```python
from build123d import *

# Parameters (mm, degrees)
F0_R     = 8.05
F1_DEPTH = 3.6
F2_R     = 6
F3_DEPTH = 6
F4_R     = 8.05
F5_DEPTH = 3.1
F6_R     = 5
F7_DEPTH = 2.5
F8_R     = 2
F9_DEPTH = 15.201


with BuildPart() as f1:
    # F0 (on Top) → F1 (new body)
    with BuildSketch(Plane.XY):
        Circle(F0_R)
    extrude(amount=F1_DEPTH)

    # F2 (on face) → F3 (join)
    with BuildSketch(Plane.XY.offset(3.6)):
        Circle(F2_R)
    extrude(amount=F3_DEPTH)

    # F4 (on face) → F5 (join)
    with BuildSketch(Plane.XY.offset(9.6)):
        Circle(F4_R)
    extrude(amount=F5_DEPTH)

    # F6 (on face) → F7 (join)
    with BuildSketch(Plane.XY.offset(12.7)):
        Circle(F6_R)
    extrude(amount=F7_DEPTH)

    # F8 (on face) → F9 (cut, through all)
    with BuildSketch(Plane(origin=(0, 0, 0), x_dir=(1, 0, 0), z_dir=(0, 0, -1))):
        Circle(F8_R)
    extrude(amount=-F9_DEPTH, mode=Mode.SUBTRACT)


solid = f1.part
```
Input: part model. Units: mm. Frame: model coordinates. A direction names the side the tool comes from. Round coordinates to 2 decimals unless told otherwise and drop trailing zeros. Loops run counter-clockwise (first coordinate to the right, second up) from the corner with the lowest first, then second, coordinate; pieces in that order, holes last. Notation, with made-up numbers: (-14, 45.25) -> (42, 45.25) arc R22 cw to (42, 61.25) -> close; hole circle Ø5 at (49, -21.75). An arc over 180 degrees is marked (long way). One line per item, written item: value.
(1) Set-up query: faces 4 (the face through (7.678, 2.418, 1.775)), 5 (the face through (-5.404, -2.944, 9.6)), 6 (the face through (-1.08, -4.88, 13.93)). Return all of +Z, -Z, +X, -X, +Y, -Y with unobstructed straight access to the full face (end or side cutting, diameter ignored); none if empty.
Geometry check:
face 4: +Z, -Z
face 5: none
face 6: +Z
(2) Section A-A (y = 0). Return the cut outline in (x, z), plus the area to 3 significant figures.
Geometry check:
outline: (-8.05, 0) -> (-2, 0) -> (-2, 15.2) -> (-5, 15.2) -> (-5, 12.7) -> (-8.05, 12.7) -> (-8.05, 9.6) -> (-6, 9.6) -> (-6, 3.6) -> (-8.05, 3.6) -> close; (2, 0) -> (8.05, 0) -> (8.05, 3.6) -> (6, 3.6) -> (6, 9.6) -> (8.05, 9.6) -> (8.05, 12.7) -> (5, 12.7) -> (5, 15.2) -> (2, 15.2) -> close
area: 144 mm2
(3) Section D-D (x = -6.5). Return the cut outline in (y, z), plus the area to 3 significant figures.
Geometry check:
outline: (-4.75, 0) -> (4.75, 0) -> (4.75, 3.6) -> (-4.75, 3.6) -> close; (-4.75, 9.6) -> (4.75, 9.6) -> (4.75, 12.7) -> (-4.75, 12.7) -> close
area: 63.6 mm2
(4) Material intervals for line 1 (Y direction, x = 0, z = 11.75); line 2 (Z direction, x = -0.25, y = 7.25); line 3 (Y direction, x = 0, z = 6), sorted ascending. Write a range as [from, to].
Geometry check:
line 1: [-8.05, -2], [2, 8.05]
line 2: [0, 3.6], [9.6, 12.7]
line 3: [-6, -2], [2, 6]
(5) Mould query, pull axis X, two halves, no side actions, for faces 1 (the face through (0, 2, 7)), 2 (the face through (-0.1, -5.3, 12.7)), 3 (the face through (7.678, 2.418, 11.128)). Classes: pulls with the +X half, pulls with the -X half, needs draft (parallel to the pull), parting line crosses it, or undercut.
Geometry check:
face 1: undercut
face 2: needs draft
face 3: parting line crosses it
(6) Pin query (flat end, axial travel): pin 1 (1.5 mm diameter, centred on y = 5.5, z = 4, fed in from +X); pin 2 (6 mm diameter, centred on x = -2, z = 7, fed in from -Y); pin 3 (2 mm diameter, centred on x = -2.5, z = 7.5, fed in from +Y). Return the tip coordinate at first contact, or that it passes through.
Geometry check:
pin 1: x = 6.41
pin 2: y = -8.03
pin 3: y = 5.81
(7) Section C-C (z = 7). Return the cut outline in (x, y).
Geometry check:
outline: circle Ø12 at (0, 0); hole circle Ø4 at (0, 0)
